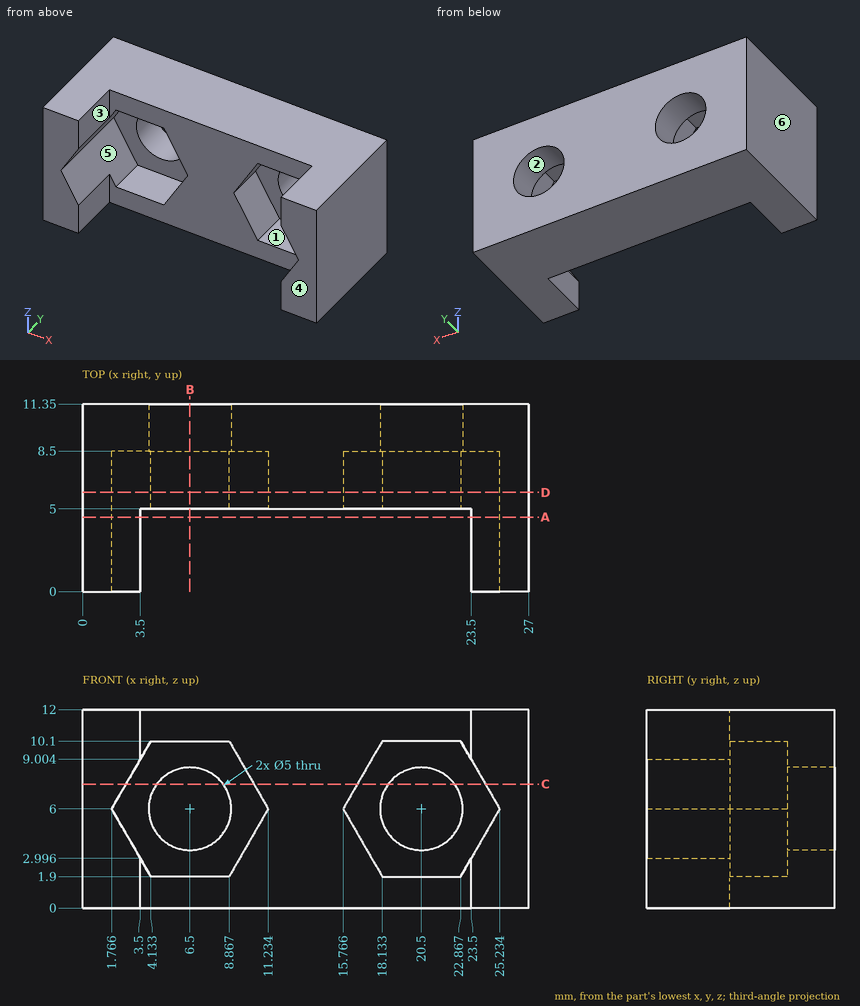
Here's the drawing with two shaded views (mm, measured from the low corner). I have some questions. A direction names the side the tool comes from. Coordinates: 2 decimals unless noted, no trailing zeros. Write each loop counter-clockwise with the first axis right and the second up, starting at its lowest first coordinate (ties: lowest second). Pieces come first, ordered by that corner, then holes.
Item 1: On a 3-axis mill with a long thin cutter (end or side, diameter ignored), from which of +Z, -Z, +X, -X, +Y, -Y can I reach the whole of each face in a straight line? I mean the marked faces 1, 2 and 3. Say none if no direction works.
Item 2: I want a section at B-B on x = 6.5. Write out the boundary of the cut face in (y, z).
Item 3: I want a section at A-A on y = 4.5. Write out the boundary of the cut face in (x, z).
Item 4: I want a section at D-D on y = 6. Write out the boundary of the cut face in (x, z).
Item 5: I want a section at C-C on z = 7.5. Write out the boundary of the cut face in (x, y).
Item 6: Will these pins go through, and if not, where does the flat tip stop? pin 1 (6.5 mm diameter, centred on x = 8, z = 4, fed in from -Y); pin 2 (4.5 mm diameter, centred on x = 6.5, z = 6, fed in from +Y); pin 3 (2.5 mm diameter, centred on x = 20, z = 4, fed in from -Y).
Item 7: If we mould it in two halves opening along X, with no side actions, what happens to the marked faces 4, 5 and 6? For each: +X half, -X half, draft (parallel to the pull), parting line (faces both ways), or undercut.
Item 8: If I drill on line 1 (X direction, y = 10.4, z = 6); line 2 (Z direction, x = 20.5, y = 9.9); line 3 (Z direction, x = 19.5, y = 7.5), over which ranges is the centre line in solid material (lowest first)?
Findings below:
1. face 1: -Y
1. face 2: +Y, -Y
1. face 3: +Z, -Z, -Y
2. outline: (5, 0) - (11.35, 0) - (11.35, 3.5) - (8.5, 3.5) - (8.5, 1.9) - (5, 1.9) - close; (5, 10.1) - (8.5, 10.1) - (8.5, 8.5) - (11.35, 8.5) - (11.35, 12) - (5, 12) - close
3. outline: (0, 0) - (3.5, 0) - (3.5, 3) - (1.77, 6) - (3.5, 9) - (3.5, 12) - (0, 12) - close; (23.5, 0) - (27, 0) - (27, 12) - (23.5, 12) - (23.5, 9) - (25.23, 6) - (23.5, 3) - close
4. outline: (0, 0) - (27, 0) - (27, 12) - (0, 12) - close; hole (1.77, 6) - (4.13, 1.9) - (8.87, 1.9) - (11.23, 6) - (8.87, 10.1) - (4.13, 10.1) - close; hole (15.77, 6) - (18.13, 1.9) - (22.87, 1.9) - (25.23, 6) - (22.87, 10.1) - (18.13, 10.1) - close
5. outline: (0, 0) - (2.63, 0) - (2.63, 8.5) - (4.5, 8.5) - (4.5, 11.35) - (0, 11.35) - close; (8.5, 8.5) - (10.37, 8.5) - (10.37, 5) - (16.63, 5) - (16.63, 8.5) - (18.5, 8.5) - (18.5, 11.35) - (8.5, 11.35) - close; (22.5, 8.5) - (24.37, 8.5) - (24.37, 0) - (27, 0) - (27, 11.35) - (22.5, 11.35) - close
6. pin 1: stops at y = 5
6. pin 2: passes through
6. pin 3: stops at y = 8.5
7. face 4: draft
7. face 5: undercut
7. face 6: -X half
8. line 1: x = 0 to 4, 9 to 18, 23 to 27
8. line 2: z = 0 to 3.5, 8.5 to 12
8. line 3: z = 0 to 1.9, 10.1 to 12
